Autodesk Inventor part; units mm, degrees
ref_plane "YZ Plane" through (0, 0, 0) normal (1, 0, 0) x (0, 1, 0)
ref_plane "XZ Plane" through (0, 0, 0) normal (0, 1, 0) x (-1, 0, 0)
ref_plane "XY Plane" through (0, 0, 0) normal (0, 0, 1) x (1, 0, 0)
sketch "Sketch1" plane through (0, 0, 0) normal (0, 0, 1) x (1, 0, 0)
  line L0 (0, 0) -> (165, 0)
  line L1 (165, 0) -> (165, 50)
  line L2 (165, 50) -> (0, 50)
  line L3 (0, 50) -> (0, 0)
  line L4 (0, 50) -> (3, 50)
  line L5 (3, 50) -> (3, 46.5)
  line L6 (3, 46.5) -> (0, 46.5)
  line L7 (0, 46.5) -> (0, 50)
  line L8 (0, 0) -> (3, 0)
  line L9 (3, 0) -> (3, 3.5)
  line L10 (3, 3.5) -> (0, 3.5)
  line L11 (0, 3.5) -> (0, 0)
  line L12 (82.5, 0) -> (82.5, 50) construction
  line L13 (162, 50) -> (162, 46.5)
  line L14 (162, 46.5) -> (165, 46.5)
  line L15 (162, 0) -> (162, 3.5)
  line L16 (162, 3.5) -> (165, 3.5)
  line L17 (44, 46.5) -> (121, 46.5) construction
  line L18 (121, 46.5) -> (121, 3.5) construction
  line L19 (121, 3.5) -> (44, 3.5) construction
  line L20 (44, 3.5) -> (44, 46.5) construction
  line L21 (53, 46.5) -> (114, 46.5)
  line L22 (114, 46.5) -> (114, 3.5)
  line L23 (114, 3.5) -> (53, 3.5)
  line L24 (53, 3.5) -> (53, 46.5)
  line L25 (3, 0) -> (0, 0)
  line L26 (0, 0) -> (0, 8)
  line L27 (0, 8) -> (3, 8)
  line L28 (3, 8) -> (3, 0)
  line L29 (0, 50) -> (3, 50)
  line L30 (3, 50) -> (3, 42)
  line L31 (3, 42) -> (0, 42)
  line L32 (0, 42) -> (0, 50)
  line L33 (0, 42) -> (3, 42)
  line L34 (3, 42) -> (3, 30)
  line L35 (3, 30) -> (0, 30)
  line L36 (0, 30) -> (0, 42)
  line L37 (3, 8) -> (0, 8)
  line L38 (0, 8) -> (0, 20)
  line L39 (0, 20) -> (3, 20)
  line L40 (3, 20) -> (3, 8)
  line L41 (165, 8) -> (162, 8)
  line L42 (162, 42) -> (165, 42)
  line L43 (162, 42) -> (162, 30)
  line L44 (162, 30) -> (165, 30)
  line L45 (165, 20) -> (162, 20)
  line L46 (162, 20) -> (162, 8)
  point P0 (1.5, 25)
  point P1 (0, 25)
  point P2 (1.5, 3.5)
  point P3 (44, 25)
  point P4 (82.5, 46.5)
  point P5 (1.5, 46.5)
  point P6 (119, 5.5)
  point P7 (119, 44.5)
  point P8 (50.5, 44.5)
  point P9 (50.5, 5.5)
  point P10 (0, 46.5)
  point P11 (0, 3.5)
  point P12 (165, 20)
  point P13 (165, 30)
  point P14 (165, 42)
  dimension "d0" = 165
  dimension "d1" = 50
  dimension "d2" = 3
  dimension "d4" = 21.5
  dimension "d5" = 21.5
  dimension "d6" = 77
  dimension "d7" = 61
  dimension "d8" = 9
  dimension "d9" = 2
  dimension "d10" = 2
  dimension "d11" = 2
  dimension "d12" = 6.5
  dimension "d13" = 2
  dimension "d34" = 8
  dimension "d35" = 8
  dimension "d36" = 12
  dimension "d37" = 12
extrude "Extrusion1" add sketch "Sketch1" along normal blind 3 contours L3 L10 L9 L0 | L9 L28 L40 L39 L3 L35 L34 L30 L5 L2 L13 L14 L1 L42 L43 L44 L45 L46 L41 L16 L15 L0 | L3 L27 L28 L10 | L15 L16 L1 L0 | L3 L6 L30 L31 | L3 L2 L5 L6 | L14 L13 L2 L1
sketch "Sketch2" plane through (0, 0, 3) normal (0, 0, 1) x (1, 0, 0)
  line L0 (53, 46.5) -> (114, 46.5)
  line L1 (44, 46.5) -> (121, 46.5)
  line L2 (121, 46.5) -> (121, 0)
  line L3 (121, 0) -> (44, 0)
  line L4 (44, 0) -> (44, 46.5)
  line L5 (165, 50) -> (0, 50)
  line L6 (0, 8) -> (0, 0)
  point P0 (50.92, 43.5)
  point P1 (50.92, 3)
  point P2 (82.5, 46.5)
  point P3 (82.5, 50)
  point P4 (113, 50)
  point P5 (3, 50)
  point P6 (44, 23.25)
  point P7 (0, 4)
  point P8 (0, 46.5)
  point P9 (0, 3.5)
  point P10 (118, 43.5)
  point P11 (118, 3)
  dimension "d17" = 77
  dimension "d18" = 3
  dimension "d19" = 3
  dimension "d20" = 3
  dimension "d28" = 6.92
hole "Hole1" at (50.92, 43.5, 3) at (50.92, 3, 3) at (118, 3, 3) at (118, 43.5, 3) direction (0, 0, -1) diameter 3 end through all
sketch "Sketch3" plane through (0, 0, 3) normal (0, 0, 1) x (1, 0, 0)
  line L0 (10, 34.5) -> (23, 34.5)
  line L1 (23, 34.5) -> (23, 15.5)
  line L2 (23, 15.5) -> (10, 15.5)
  line L3 (10, 15.5) -> (10, 34.5)
  line L4 (0, 8) -> (0, 0) construction
  line L5 (144.7, 31.65) -> (155, 31.65)
  line L6 (155, 31.65) -> (155, 18.35)
  line L7 (155, 18.35) -> (144.7, 18.35)
  line L8 (144.7, 18.35) -> (144.7, 31.65)
  line L9 (165, 20) -> (165, 30)
  line L10 (0, 30) -> (0, 20)
  point P0 (10, 25)
  point P1 (0, 46.5)
  point P2 (165, 25)
  point P3 (0, 25)
  point P4 (144.7, 25)
  dimension "d29" = 19
  dimension "d30" = 13
  dimension "d31" = 10
  dimension "d38" = 10.3
  dimension "d39" = 13.3
  dimension "d40" = 10
extrude "Extrusion2" cut sketch "Sketch3" against normal blind 10
properties part number "pantallaSoport"
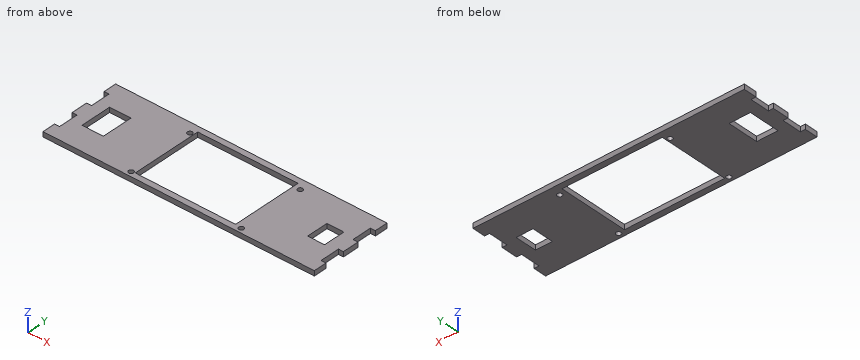
Geometry check sheet. Reference: the model listing, model coordinates, mm. Coordinates: 2 decimals unless noted, no trailing zeros. Loops run counter-clockwise (first coordinate to the right, second up) from the corner with the lowest first, then second, coordinate; pieces in that order, holes last. Notation, with made-up numbers: (68, 35.25) - (86, 35.25) arc R24 ccw to (86, 50.25) - close; hole circle Ø6 at (20.5, 22). An arc over 180 degrees is marked (long way). Use one line per item in the form item = value. Start each with the question number.
Item 1: Section check B-B, the plane x = 82.5. Enter the section's corners in (y, z), and give its area (3 significant figures).
Item 2: Thickness scan on probe 1 along X at (y, z) = (16, 0.4); probe 2 along X at (y, z) = (3, 0.7); probe 3 along Y at (x, z) = (50.92, 2.05). Record the ranges inside material, lowest first.
Item 3: Gauge pin test, flat ends, axial feed: pin 1 (1.5 mm diameter, centred on y = 14, z = 1.5, fed in from +X); pin 2 (1 mm diameter, centred on y = 15.5, z = 2, fed in from -X). Record the tip position at first contact, or that the pin passes through.
Item 4: Section check C-C, the plane x = 50.92. Enter the section's corners in (y, z), and give its area (3 significant figures).
Item 5: Section check A-A, the plane y = 38. Enter the section's corners in (x, z).
Item 6: Section check D-D, the plane z = 1.3. Give the number of separate pieces and of enclosed holes in the cut face, and give its area (3 significant figures).
Computed:
q1.outline = (0, 0) - (3.5, 0) - (3.5, 3) - (0, 3) - close; (46.5, 0) - (50, 0) - (50, 3) - (46.5, 3) - close
q1.area = 21.0 mm2
q2.probe_1 = 3 to 10, 23 to 53, 114 to 162
q2.probe_2 = 0 to 49.42, 52.42 to 116.5, 119.5 to 165
q2.probe_3 = 0 to 1.5, 4.5 to 42, 45 to 50
q3.pin_1 = 162
q3.pin_2 = 3
q4.outline = (0, 0) - (1.5, 0) - (1.5, 3) - (0, 3) - close; (4.5, 0) - (42, 0) - (42, 3) - (4.5, 3) - close; (45, 0) - (50, 0) - (50, 3) - (45, 3) - close
q4.area = 132 mm2
q5.outline = (3, 0) - (53, 0) - (53, 3) - (3, 3) - close; (114, 0) - (162, 0) - (162, 3) - (114, 3) - close
q6.separate_pieces = 1
q6.enclosed_holes = 7
q6.area = 5,070 mm2
